from build123d import *

# Parameters (mm, degrees)
BASE_EXTRUDE_DEPTH = 101.6
SLOT_DEPTH         = 145.160282621
LPATTERN1_COUNT    = 2
LPATTERN1_PITCH    = 50.8


with BuildPart() as part:
    # Sketch1 → Base-Extrude (new body)
    with BuildSketch(Plane.XY):
        with BuildLine():
            Line((-20.6375, 39.6875), (-20.6375, -35.4076))
            ThreePointArc((-20.6375, -35.4076), (-19.848914298, -37.311414298), (-17.9451, -38.1))
            Line((-17.9451, -38.1), (17.9451, -38.1))
            ThreePointArc((17.9451, -38.1), (19.848914298, -37.311414298), (20.6375, -35.4076))
            Line((20.6375, -35.4076), (20.6375, 39.6875))
            ThreePointArc((20.6375, 39.6875), (15.875, 44.45), (11.1125, 39.6875))
            Line((11.1125, 39.6875), (11.1125, 38.65245))
            ThreePointArc((11.1125, 38.65245), (12.4587, 37.30625), (13.8049, 38.65245))
            Line((13.8049, 38.65245), (13.8049, 39.6875))
            ThreePointArc((13.8049, 39.6875), (15.875, 41.7576), (17.9451, 39.6875))
            Line((17.9451, 39.6875), (17.9451, -35.4076))
            Line((17.9451, -35.4076), (-17.9451, -35.4076))
            Line((-17.9451, -35.4076), (-17.9451, 39.6875))
            ThreePointArc((-17.9451, 39.6875), (-15.875, 41.7576), (-13.8049, 39.6875))
            Line((-13.8049, 39.6875), (-13.8049, 38.65245))
            ThreePointArc((-13.8049, 38.65245), (-12.4587, 37.30625), (-11.1125, 38.65245))
            Line((-11.1125, 38.65245), (-11.1125, 39.6875))
            ThreePointArc((-11.1125, 39.6875), (-15.875, 44.45), (-20.6375, 39.6875))
        make_face()
    extrude(amount=BASE_EXTRUDE_DEPTH)

    # Sketch2 → Slot (cut, through all)
    with BuildSketch(Plane(origin=(-0.560706402, -38.1, -14.668313098), x_dir=(1, 0, 0), z_dir=(0, -1, 0))):
        with BuildLine():
            Line((7.704456402, 51.974563098), (7.704456402, 37.687063098))
            ThreePointArc((7.704456402, 37.687063098), (0.560706402, 30.543313098), (-6.583043598, 37.687063098))
            Line((-6.583043598, 37.687063098), (-6.583043598, 51.974563098))
            ThreePointArc((-6.583043598, 51.974563098), (0.560706402, 59.118313098), (7.704456402, 51.974563098))
        make_face()
    slot = extrude(amount=-SLOT_DEPTH, mode=Mode.SUBTRACT)

    # LPattern1: Slot ×2
    with Locations(*[(0, 0, i * LPATTERN1_PITCH) for i in range(1, LPATTERN1_COUNT)]):
        add(slot, mode=Mode.SUBTRACT)


solid = part.part
Geometry: final body of the model. Coordinates: model frame, mm. A direction names the side the tool comes from. Round coordinates to 2 decimals unless told otherwise and drop trailing zeros. Order: outer loops, then holes, each group sorted by start corner. A loop starts at its lowest first (then second) coordinate and runs counter-clockwise, first axis right, second up. Notation, with made-up numbers: (68, 17) - (94, 17) arc R14 ccw to (94, 40) - close; hole circle Ø10 at (-5, 15). An arc over 180 degrees is marked (long way). Write each question's results on one line, items separated by ' | '.
Item 1: Material intervals for line 1 along X through (y, z) = (21, 67); line 2 along Y through (x, z) = (16, 61.5); line 3 along Y through (x, z) = (-14.5, 42), sorted ascending. Write a range as [from, to].
Completed:
line 1: [-20.64, -17.95], [17.95, 20.64] | line 2: [-38.1, -35.41], [41.75, 44.45] | line 3: [-38.1, -35.41], [41.23, 44.25]
Item 2: Section B-B, the plane x = 0. Return the cut outline in (y, z) (3 decimals).
Completed:
outline: (-38.1, 0) - (-35.408, 0) - (-35.408, 15.875) - (-38.1, 15.875) - close; (-38.1, 44.45) - (-35.408, 44.45) - (-35.408, 66.675) - (-38.1, 66.675) - close; (-38.1, 95.25) - (-35.408, 95.25) - (-35.408, 101.6) - (-38.1, 101.6) - close
Item 3: Mould query, pull axis Z, two halves, no side actions, for faces 4 (the cylindrical face through (-15.77, 44.45, 50.09)), 5 (the flat face through (18.2, -2.7, 0)), 6 (the flat face through (-7.144, -37, 81)), 7 (the cylindrical face through (-0.16, -36.77, 95.25)). Classes: pulls with the +Z half, pulls with the -Z half, needs draft (parallel to the pull), parting line crosses it, or undercut.
Completed:
face 4: needs draft | face 5: pulls with the -Z half | face 6: undercut | face 7: undercut
Item 4: Reachability of faces 1 (the cylindrical face through (0.157, -36.773, 15.877)), 2 (the flat face through (-17.945, 2, 50)), 3 (the cylindrical face through (15.98, 44.45, 50.09)) from +Z, -Z, +X, -X, +Y, -Y: full face, straight path, thin tool, end or side. Return the list, or none.
Completed:
face 1: +Y, -Y | face 2: +Z, -Z | face 3: +Z, -Z, +Y
Item 5: Section D-D, the plane z = 48.5. Return the cut outline in (x, y) (1 decimal), and give its area (3 significant figures).
Completed:
outline: (-20.6, -35.4) arc R2.7 ccw to (-17.9, -38.1) - (17.9, -38.1) arc R2.7 ccw to (20.6, -35.4) - (20.6, 39.7) arc R4.8 ccw to (11.1, 39.7) - (11.1, 38.7) arc R1.3 ccw to (13.8, 38.7) - (13.8, 39.7) arc R2.1 cw to (17.9, 39.7) - (17.9, -35.4) - (-17.9, -35.4) - (-17.9, 39.7) arc R2.1 cw to (-13.8, 39.7) - (-13.8, 38.7) arc R1.3 ccw to (-11.1, 38.7) - (-11.1, 39.7) arc R4.8 ccw to (-20.6, 39.7) - close | area: 581 mm^2
Item 6: First-contact query: pin 1 Ø11 at (x, z) = (4, 43.5) entering from +Y; pin 2 Ø0.8 at (y, z) = (-36.5, 28) entering from +X; pin 3 Ø2 at (y, z) = (-37, 79) entering from -X. Flat tips, straight axial feed; report the tip coordinate or a pass-through.
Completed:
pin 1: y = -35.41 | pin 2: x = 20.55 | pin 3: x = -20.57
Item 7: Section A-A, the plane y = 8. Return the cut outline in (x, z), and give its area (3 significant figures).
Completed:
outline: (-20.64, 0) - (-17.95, 0) - (-17.95, 101.6) - (-20.64, 101.6) - close; (17.95, 0) - (20.64, 0) - (20.64, 101.6) - (17.95, 101.6) - close | area: 547 mm^2
Item 8: Section C-C, the plane z = 75.5. Return the cut outline in (x, y) (1 decimal).
Completed:
outline: (-20.6, -35.4) arc R2.7 ccw to (-17.9, -38.1) - (-7.1, -38.1) - (-7.1, -35.4) - (-17.9, -35.4) - (-17.9, 39.7) arc R2.1 cw to (-13.8, 39.7) - (-13.8, 38.7) arc R1.3 ccw to (-11.1, 38.7) - (-11.1, 39.7) arc R4.8 ccw to (-20.6, 39.7) - close; (7.1, -38.1) - (17.9, -38.1) arc R2.7 ccw to (20.6, -35.4) - (20.6, 39.7) arc R4.8 ccw to (11.1, 39.7) - (11.1, 38.7) arc R1.3 ccw to (13.8, 38.7) - (13.8, 39.7) arc R2.1 cw to (17.9, 39.7) - (17.9, -35.4) - (7.1, -35.4) - close
